from build123d import *

# Parameters (mm, degrees)
PAD001_DEPTH         = 4.5
FILLET_R             = 4.4
CHAMFER_1_SIZE2      = 2
CHAMFER_1_SIZE       = 1
CHAMFER_2_SIZE2      = 2
CHAMFER_2_SIZE       = 1
CHAMFER001_SIZE      = 2
PAD002_DEPTH         = 4.5
SKETCH006_R          = 2.5
POCKET001_DEPTH      = 36.001
POCKET001_DEPTH_BACK = 36.001


with BuildPart() as part:
    # Sketch004 → Pad001 (new body, symmetric)
    with BuildSketch(Plane.YZ):
        Polygon((-31, 5.5), (-31, -14), (0, -31.897858), (0, -35.558112), (-3.660254, -35.558112), (-36, -16.886751), (-36, 14.5), (-25, 14.5), (-25, 5.5), align=None)
    pad001 = extrude(amount=PAD001_DEPTH, both=True)

    # Mirrored: Pad001 across Sketch004 V_Axis
    add(pad001.mirror(Plane(origin=(0, 0, 0), x_dir=(1, 0, 0), z_dir=(0, 1, 0))))

    # Fillet
    fillet_edges = [part.edges().sort_by_distance(p)[0] for p in [
        (-4.5, 28, 5.5),
        (-4.5, 30.5, 14.5),
        (4.5, 28, 5.5),
        (-4.5, -28, 5.5),
        (-4.5, -30.5, 14.5),
        (4.5, -30.5, 14.5),
        (4.5, 30.5, 14.5),
        (4.5, -28, 5.5),
    ]]
    fillet(fillet_edges, radius=FILLET_R)

    # Chamfer 1
    chamfer_1_edges = [part.edges().sort_by_distance(p)[0] for p in [
        (-3.21127, 25, 13.21127),
    ]]
    chamfer_1_side = part.faces().sort_by_distance((0, 25, 10))[0]
    chamfer(chamfer_1_edges, length=CHAMFER_1_SIZE, length2=CHAMFER_1_SIZE2, reference=chamfer_1_side)

    # Chamfer 2
    chamfer_2_edges = [part.edges().sort_by_distance(p)[0] for p in [
        (-3.21127, -25, 13.21127),
    ]]
    chamfer_2_side = part.faces().sort_by_distance((0, -25, 10))[0]
    chamfer(chamfer_2_edges, length=CHAMFER_2_SIZE, length2=CHAMFER_2_SIZE2, reference=chamfer_2_side)

    # Chamfer001
    chamfer001_edges = [part.edges().sort_by_distance(p)[0] for p in [
        (0, 0, -31.897858),
    ]]
    chamfer(chamfer001_edges, length=CHAMFER001_SIZE)

    # Sketch005 → Pad002 (join, symmetric)
    with BuildSketch(Plane.YZ):
        Polygon((-34, -12), (34, -12), (34, -17), (4, -17), (0, -14), (-4, -17), (-34, -17), align=None)
    extrude(amount=PAD002_DEPTH, both=True)

    # Sketch006 → Pocket001 (cut, two sides)
    with BuildSketch(Plane.XZ) as pocket001_sk:
        with Locations((0, 10)):
            Circle(SKETCH006_R)
    extrude(amount=-POCKET001_DEPTH, mode=Mode.SUBTRACT)
    extrude(pocket001_sk.sketch, amount=POCKET001_DEPTH_BACK, mode=Mode.SUBTRACT)


solid = part.part
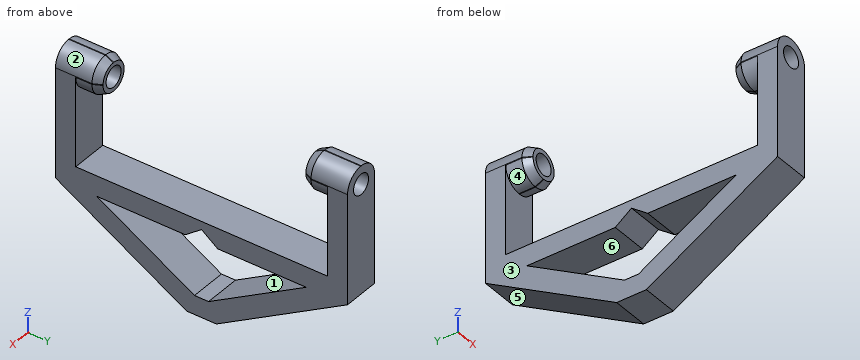
Verification items for the finished model (mm, model axes). Face numbers are marked on the shaded views. A direction names the side the tool comes from. Round coordinates to 2 decimals unless told otherwise and drop trailing zeros. Order: outer loops, then holes, each group sorted by start corner. A loop starts at its lowest first (then second) coordinate and runs counter-clockwise, first axis right, second up.
1. Section check A-A on z = -5. Record the cut outline in (x, y), then the cut area to 3 significant figures.
Final values:
outline: (-4.5, -36) - (4.5, -36) - (4.5, -31) - (-4.5, -31) - close; (-4.5, 31) - (4.5, 31) - (4.5, 36) - (-4.5, 36) - close
area: 90.0 mm2
2. Thickness scan on L1, parallel to X at y = -32, z = 10; L2, parallel to Y at x = 3.25, z = 10; L3, parallel to Y at x = -2.5, z = 1.5. Record the ranges inside material, lowest first.
Final values:
L1: x = -4.5 to -2.5, 2.5 to 4.5
L2: y = -36 to -25, 25 to 36
L3: y = -36 to -31, 31 to 36
3. Access from +Z, -Z, +X, -X, +Y, -Y to the whole of each face (thin tool, end or side, straight path). Record for the marked faces 4, 5 and 6.
Final values:
face 4: -X
face 5: -Z, +X, -X, +Y
face 6: +X, -X
4. Section check B-B on y = 15.5. Record the cut outline in (x, z), then the cut area to 3 significant figures.
Final values:
outline: (-4.5, -28.72) - (4.5, -28.72) - (4.5, -22.95) - (-4.5, -22.95) - close; (-4.5, -17) - (4.5, -17) - (4.5, -12) - (-4.5, -12) - close
area: 97.0 mm2
5. Release check for a two-part mould opening along Z. For the marked faces 1, 2 and 3 record: +Z half, -Z half, draft (parallel to the pull), parting line (faces both ways), or undercut.
Final values:
face 1: undercut
face 2: +Z half
face 3: draft
6. Go/stop test with flat-tipped pins: P1, Ø4.5, axis at x = 0, z = 10, coming from the +Y side; P2, Ø2.5, axis at x = 0.5, y = 3, coming from the +Z side; P3, Ø2.5, axis at x = 0.5, y = 13, coming from the -Z side; P4, Ø2, axis at x = -1.5, z = -28.5, coming from the -Y side. Record where each tip stops, or that it passes through.
Final values:
P1: passes through
P2: stops at z = -12
P3: stops at z = -30.89
P4: stops at y = -17.62
